The model under review builds one solid part; all positions refer to its coordinate system, in mm. A direction names the side the tool comes from. Coordinates: 2 decimals unless noted, no trailing zeros. Order: outer loops, then holes, each group sorted by start corner. A loop starts at its lowest first (then second) coordinate and runs counter-clockwise, first axis right, second up.
Autodesk Inventor part; units mm, degrees
ref_plane "YZ Plane" through (0, 0, 0) normal (1, 0, 0) x (0, 1, 0)
ref_plane "XZ Plane" through (0, 0, 0) normal (0, 1, 0) x (-1, 0, 0)
ref_plane "XY Plane" through (0, 0, 0) normal (0, 0, 1) x (1, 0, 0)
sketch "Эскиз1" plane through (0, 0, 0) normal (0, 1, 0) x (-1, 0, 0)
  line L0 (17, -52.5) -> (-17, -52.5)
  line L1 (-17, -52.5) -> (-17, 52.5)
  line L2 (-17, 52.5) -> (17, 52.5)
  line L3 (17, 52.5) -> (17, -52.5)
  line L4 (17, -52.5) -> (-17, 52.5) construction
  line L5 (-17, -52.5) -> (17, 52.5) construction
  point P0 (0, 0)
  dimension "d0" = 105
  dimension "d1" = 34
extrude "Выдавливание1" add sketch "Эскиз1" along normal blind 27
fillet "Сопряжение1" radius 4 12 edges at (17, 0, 0) (-17, 0, 0) (-17, 27, 0) (17, 27, 0) (0, 27, 52.5) (17, 13.5, 52.5) (0, 0, 52.5) (-17, 13.5, 52.5) (17, 13.5, -52.5) (0, 0, -52.5) (-17, 13.5, -52.5) (0, 27, -52.5)
sketch "Эскиз2" plane through (-13, 4, 52.5) normal (0, 0, 1) x (1, 0, 0)
  line L0 (26, 23) -> (0, 23)
  circle A0 centre (-1.8428, 14.4631) radius 2.25
  circle A1 centre (-1.8428, 4.066) radius 2.25
  circle A2 centre (-3.2811, 6.8739) radius 0.75
  circle A3 centre (-3.2811, 8.3904) radius 0.75
  circle A4 centre (-3.2811, 10.0466) radius 0.75
  circle A5 centre (-3.2811, 11.6568) radius 0.75
  point P0 (13, -4)
  dimension "d5" = 4.5
  dimension "d6" = 4.5
  dimension "d7" = 1.5
  dimension "d8" = 1.5
  dimension "d9" = 1.5
  dimension "d10" = 1.5
extrude "Выдавливание2" add sketch "Эскиз2" along normal blind 15.25 and the other way blind 4
properties part number "Аккамулятор" material "Пластик ПАЭК"
(1) We need section B-B, the plane x = -1.5. Write out the cut boundary in (y, z), and give its area (3 significant figures).
A:
outline: (0, -48.5) arc R4 ccw to (4, -52.5) - (23, -52.5) arc R4 ccw to (27, -48.5) - (27, 48.5) arc R4 ccw to (23, 52.5) - (4, 52.5) arc R4 ccw to (0, 48.5) - close
area: 2,820 mm2
(2) We need section A-A, the plane z = 3.5. Write out the cut boundary in (x, y).
A:
outline: (-17, 4) arc R4 ccw to (-13, 0) - (13, 0) arc R4 ccw to (17, 4) - (17, 23) arc R4 ccw to (13, 27) - (-13, 27) arc R4 ccw to (-17, 23) - close
(3) Draft analysis for pull direction Y (two halves, no side actions). For faces 1 (the face through (0, 0, 1)), 2 (the face through (-17.09, 7.97, 60.13)), 3 (the face through (0.182, 25.797, -51.359)), state which applies: released by +Y, released by -Y, zero draft, split by the parting line, or undercut.
A:
face 1: released by -Y
face 2: undercut
face 3: released by +Y
(4) We need section C-C, the plane z = 50.5. Write out the cut boundary in (x, y).
A:
outline: (-16.46, 4) arc R3.46 ccw to (-13, 0.54) - (13, 0.54) arc R3.46 ccw to (16.46, 4) - (16.46, 23) arc R3.46 ccw to (13, 26.46) - (-13, 26.46) arc R3.46 ccw to (-16.46, 23) - (-16.46, 20.02) arc R2.25 ccw to (-16.46, 16.9) - (-16.46, 16.38) arc R0.75 ccw to (-16.46, 14.93) - (-16.46, 14.77) arc R0.75 ccw to (-16.46, 13.32) - (-16.46, 13.12) arc R0.75 ccw to (-16.46, 11.66) - (-16.46, 11.6) arc R0.75 ccw to (-16.46, 10.15) - (-16.46, 9.63) arc R2.25 ccw to (-16.46, 6.51) - close
(5) For pin 1 Ø2 at (y, z) = (20, 22.5) entering from -X; pin 2 Ø1.5 at (x, y) = (-8.5, 14.5) entering from +Z, all flat-tipped, find the tip position at first contact; note any pin that passes through.
A:
pin 1: stops at x = -17
pin 2: stops at z = 52.5
(6) Machinability: for faces 4 (the face through (-17.09, 18.56, 60.4)), 5 (the face through (15.859, 13.633, -51.297)), which of the approach directions +Z, -Z, +X, -X, +Y, -Y give a long, thin tool a straight path to every point of the face, cutting with its end or side? Answer none if there is none.
A:
face 4: +Z
face 5: -Z, +X, +Y, -Y
(7) Wall thickness on probe 1 along Z at (x, y) = (0.5, 10.75); probe 2 along X at (y, z) = (18.75, 17.5); probe 3 along Y at (x, z) = (-15, -13): over which ranges is each line inside the solid? List them lowest first.
A:
probe 1: z = -52.5 to 52.5
probe 2: x = -17 to 17
probe 3: y = 0.54 to 26.46
